Part print with two shaded views. Sizes in mm from the minimum x, y, z corner. A direction names the side the tool comes from. Round coordinates to 2 decimals unless told otherwise and drop trailing zeros. Write each loop counter-clockwise with the first axis right and the second up, starting at its lowest first coordinate (ties: lowest second). Pieces come first, ordered by that corner, then holes. Notation, with made-up numbers: (40, -36) -> (70, -36) arc R30 ccw to (70, 3) -> close; hole circle Ø8 at (41.25, 55). An arc over 180 degrees is marked (long way). Answer as CSV lines item,"result".
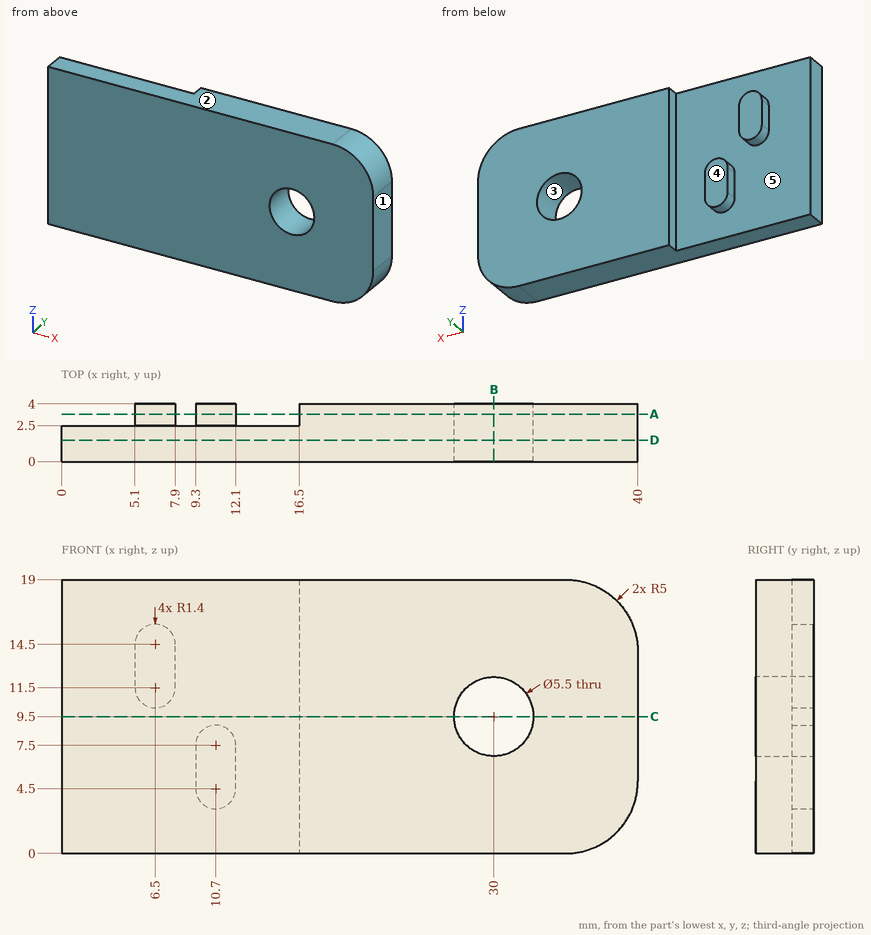
1. Mould opens along Z. For the marked faces 1, 2 and 3 say: +Z half, -Z half, draft (parallel to the pull), parting line (faces both ways), or undercut.
Results found:
face 1,"draft"
face 2,"+Z half"
face 3,"undercut"
2. Which spindle directions (+Z, -Z, +X, -X, +Y, -Y) get a long thin tool onto all of the face, cutting with end or side? Do the marked faces 4 and 5. Say none if no direction does.
Results found:
face 4,"+Z, -Z, +X, -X, +Y"
face 5,"+Y"
3. Cut at D-D, the plane y = 1.5. Write the cut outline in (x, z).
Results found:
outline,"(0, 0) -> (35, 0) arc R5 ccw to (40, 5) -> (40, 14) arc R5 ccw to (35, 19) -> (0, 19) -> close; hole circle Ø5.5 at (30, 9.5)"
4. Cut at C-C, the plane z = 9.5. Write the cut outline in (x, y).
Results found:
outline,"(0, 0) -> (27.25, 0) -> (27.25, 4) -> (16.5, 4) -> (16.5, 2.5) -> (0, 2.5) -> close; (32.75, 0) -> (40, 0) -> (40, 4) -> (32.75, 4) -> close"
5. Probe line 1 along X through (y, z) = (2.4, 9.5); line 2 along X through (y, z) = (2.75, 9.5); line 3 along Y through (x, z) = (2, 16.5). List the from-to ranges inside material, lowest first.
Results found:
line 1,"x = 0 to 27.25, 32.75 to 40"
line 2,"x = 16.5 to 27.25, 32.75 to 40"
line 3,"y = 0 to 2.5"
6. Cut at B-B, the plane x = 30. Write the cut outline in (y, z).
Results found:
outline,"(0, 0) -> (4, 0) -> (4, 6.75) -> (0, 6.75) -> close; (0, 12.25) -> (4, 12.25) -> (4, 19) -> (0, 19) -> close"
7. Cut at A-A, the plane y = 3.3. Write the cut outline in (x, z), then the cut area to 3 significant figures.
Results found:
outline,"(5.1, 11.5) arc R1.4 ccw to (7.9, 11.5) -> (7.9, 14.5) arc R1.4 ccw to (5.1, 14.5) -> close; (9.3, 4.5) arc R1.4 ccw to (12.1, 4.5) -> (12.1, 7.5) arc R1.4 ccw to (9.3, 7.5) -> close; (16.5, 0) -> (35, 0) arc R5 ccw to (40, 5) -> (40, 14) arc R5 ccw to (35, 19) -> (16.5, 19) -> close; hole circle Ø5.5 at (30, 9.5)"
area,"441 mm2"
8. Drop flat-ended pins along their axis: pin 1 Ø1 at (y, z) = (2, 10) entering from -X; pin 2 Ø1.6 at (y, z) = (3.5, 12.5) entering from -X; pin 3 Ø0.8 at (y, z) = (3.5, 6) entering from -X; pin 4 Ø2 at (x, z) = (15, 14) entering from +Y. Give the stop position or say it passes through.
Results found:
pin 1,"stops at x = 0"
pin 2,"stops at x = 5.1"
pin 3,"stops at x = 9.3"
pin 4,"stops at y = 2.5"
